Source: CAD feature listing. Evaluate the final solid. Frame: model axes, mm. A direction names the side the tool comes from. Give positions to 0.01 mm unless a question says otherwise; leave off trailing zeros. Loops run counter-clockwise (first coordinate to the right, second up) from the corner with the lowest first, then second, coordinate; pieces in that order, holes last. Notation, with made-up numbers: M 72.5,52.5 L 114.5,52.5 A27 cw 114.5,70.5 Z; hole C 10.25,86.25 d3. An arc over 180 degrees is marked long. Answer in a Markdown table with one row per item.
```python
from build123d import *

# Parameters (mm, degrees)
F1_DEPTH = 63.5
F2_DEPTH = 25.4
F3_DEPTH = 7.9375
F0_W     = 34.8576607108
F0_H     = 28.575
F5_R     = 6.35


with BuildPart() as f1:
    # F0 (on Front) → F1 (new body, symmetric)
    with BuildSketch(Plane.XZ):
        Polygon((41.275, -9.525), (41.275, 9.525), (22.225, 9.525), (-41.275, 9.525), (-41.275, -9.525), align=None)
    extrude(amount=F1_DEPTH, both=True)

    # F0 (on Front) → F2 (join, symmetric)
    with BuildSketch(Plane.XZ):
        with BuildLine():
            Line((22.225, 9.525), (41.275, 9.525))
            Line((41.275, 9.525), (41.275, 27.0002))
            ThreePointArc((41.275, 27.0002), (45.9246798487, 38.2255201513), (57.15, 42.8752))
            Line((57.15, 42.8752), (60.325, 42.8752))
            Line((60.325, 42.8752), (60.325, 61.9252))
            Line((60.325, 61.9252), (57.15, 61.9252))
            add(Edge.make_bspline(
                [(56.1489330391, 61.9108500933), (56.4820916487, 61.9163585196), (56.8157824233, 61.9211427182), (57.15, 61.9252)],
                knots=[110.8524490967, 110.8524490967, 110.8524490967, 110.8524490967, 111.5045361635, 111.5045361635, 111.5045361635, 111.5045361635], degree=3))
            ThreePointArc((56.1489330391, 61.9108500933), (32.102865547, 51.3394004942), (22.225, 27.0002))
            Line((22.225, 27.0002), (22.225, 9.525))
        make_face()
    extrude(amount=F2_DEPTH, both=True)

    # F0 (on Front) → F3 (join, symmetric)
    with BuildSketch(Plane.XZ):
        with BuildLine():
            Line((-41.275, 9.525), (22.225, 9.525))
            Line((22.225, 9.525), (22.225, 27.0002))
            ThreePointArc((22.225, 27.0002), (32.102865547, 51.3394004942), (56.1489330391, 61.9108500933))
            add(Edge.make_bspline(
                [(-41.275, 9.525), (-41.7436731397, 39.1087358459), (-0.4868287897, 60.9744375078), (56.1489330391, 61.9108500933)],
                knots=[0, 0, 0, 0, 110.8524490967, 110.8524490967, 110.8524490967, 110.8524490967], degree=3))
        make_face()
    extrude(amount=F3_DEPTH, both=True)

    # F0 (on Front) → F4 (revolve)
    with BuildSketch(Plane.XZ):
        with Locations((93.6961696446, 52.3875)):
            Rectangle(F0_W, F0_H)
    revolve(axis=Axis((76.2673392892, 0, 52.3875), (0, 0, 1)))

    # F5
    f5_edges = [f1.edges().sort_by_distance(p)[0] for p in [
        (-41.275, -63.5, 0),
        (41.275, -63.5, 0),
        (41.275, 63.5, 0),
        (-41.275, 63.5, 0),
    ]]
    fillet(f5_edges, radius=F5_R)


solid = f1.part
```
1) Set-up query: faces 1 (the flat face through (79, 0, 38.1)), 2 (the flat face through (22.225, 17, 18)), 3 (the flat face through (37, -25.4, 36)), 4 (the flat face through (-41.275, -1, 0)). Return all of +Z, -Z, +X, -X, +Y, -Y with unobstructed straight access to the full face (end or side cutting, diameter ignored); none if empty.
Reply:
| item | result |
|---|---|
| face 1 | -Z, +X, +Y, -Y |
| face 2 | +Z, -X, +Y |
| face 3 | +Z, -X, -Y |
| face 4 | +Z, -Z, -X, +Y, -Y |
2) Pin query (flat end, axial travel): pin 1 Ø15 at (x, z) = (42.5, 28) entering from -Y; pin 2 Ø2 at (x, z) = (4, 12.5) entering from -Y; pin 3 Ø14 at (y, z) = (-19.5, 22.5) entering from -X (3 decimals). Return the tip coordinate at first contact, or that it passes through.
Reply:
| item | result |
|---|---|
| pin 1 | stops at y = -25.4 |
| pin 2 | stops at y = -7.94 |
| pin 3 | stops at x = 22.225 |
3) Material intervals for L1, parallel to X at y = -4, z = 7.5 (3 decimals); L2, parallel to Y at x = 41.5, z = 45; L3, parallel to X at y = -8, z = 12.5 (3 decimals), sorted ascending.
Reply:
| item | result |
|---|---|
| L1 | x = -41.275 to 41.275 |
| L2 | y = -25.4 to 25.4 |
| L3 | x = 22.225 to 41.275 |
4) Section A-A, the plane y = -41. Return loops of the section in (x, z) (3 decimals), then the cut area to 3 significant figures.
Reply:
| item | result |
|---|---|
| outline | M -41.275,-9.525 L 41.275,-9.525 L 41.275,9.525 L -41.275,9.525 Z |
| area | 1,570 mm² |
5) Pull-direction query (Z, two-part tool) for faces 5 (the flat face through (-1, -1, -9.525)), 6 (the cylindrical face through (-39.464, -61.59, -0.133)), 7 (the cylindrical face through (27.705, 16.547, 45.782)); classes: released by +Z, released by -Z, zero draft, split by the parting line, or undercut.
Reply:
| item | result |
|---|---|
| face 5 | released by -Z |
| face 6 | zero draft |
| face 7 | released by +Z |
